Read the model definition and answer for the solid it produces. Units are mm, in the model's axes. A direction names the side the tool comes from. Coordinates: 2 decimals unless noted, no trailing zeros. Write each loop counter-clockwise with the first axis right and the second up, starting at its lowest first coordinate (ties: lowest second). Pieces come first, ordered by that corner, then holes.
(1) Find the intervals of material crossed by probe 1 along Y at (x, z) = (0, 3); probe 2 along Z at (x, y) = (3, -16); probe 3 along X at (y, z) = (1.5, 1), in increasing order.
(2) The mould has two halves that part along Y. Classify faces 4 (the cylindrical face through (-0.54, -2.44, 4.93)), 5 (the flat face through (9.737, 4.326, 5.988)), 6 (the flat face through (-0.3, -11.6, 5.7)): +Y half, -Y half, draft (parallel to the pull), parting line (faces both ways), or undercut.
(3) Which of the six approach directions +Z, -Z, +X, -X, +Y, -Y give full straight-line access (tool end or side, diameter ignored) to faces 1 (the flat face through (4.326, -9.737, 5.988)), 2 (the flat face through (4.364, 9.311, 3.982)), 3 (the flat face through (-4.364, -9.311, 3.982))?
(4) Section A-A on z = 7.25 is taken. Write down the section's boundary in (x, y), then the cut area to 3 significant figures.
(5) Section B-B on x = -5 is taken. Write down the section's boundary in (y, z), then the cut area to 3 significant figures.
(6) Given pin 1 (3 mm diameter, centred on x = 8.5, z = 6, fed in from -Y); pin 2 (1 mm diameter, centred on y = 8.5, z = 3, fed in from +X), each flat-ended and moving along its own axis, determine where each tip first touches the part or whether it passes through.
(7) Section C-C on x = -11 is taken. Write down the section's boundary in (y, z).
from build123d import *

# Parameters (mm, degrees)
SKETCH2_R           = 5.5
SKETCH2_R_2         = 2.5
BOSS_EXTRUDE1_DEPTH = 10
BOSS_EXTRUDE2_DEPTH = 0.75
CIRPATTERN1_COUNT   = 4


with BuildPart() as part:
    # Sketch2 → Boss-Extrude1 (new body)
    with BuildSketch(Plane.XY):
        Circle(SKETCH2_R)
        Circle(SKETCH2_R_2, mode=Mode.SUBTRACT)
    extrude(amount=BOSS_EXTRUDE1_DEPTH)

    # Sketch4 → Boss-Extrude2 (add, symmetric)
    with BuildSketch(Plane(origin=(0, -1.095927867, 4.746985116), x_dir=(0, 0.9743700647852367, 0.22495105434385892), z_dir=(0, 0.22495105434385892, -0.9743700647852367))):
        with BuildLine():
            Line((5.562035005, 4.289362297), (5.562035005, 15.338741246))
            ThreePointArc((5.562035005, 15.338741246), (1.102910343, 19.797865908), (-3.356214318, 15.338741246))
            Line((-3.356214318, 15.338741246), (-3.356214318, 3.072229714))
            ThreePointArc((-3.356214318, 3.072229714), (-1.450852963, 3.954597536), (0.520369242, 3.231231872))
            ThreePointArc((0.520369242, 3.231231872), (3.26034811, 2.716133916), (5.562035005, 4.289362297))
        make_face()
    boss_extrude2 = extrude(amount=BOSS_EXTRUDE2_DEPTH, both=True)

    # CirPattern1: Boss-Extrude2 ×4 about axis
    cirpattern1_axis = Axis((0, 0, 0), (0, 0, 1))
    for i in range(1, CIRPATTERN1_COUNT):
        add(boss_extrude2.rotate(cirpattern1_axis, i * 360 / CIRPATTERN1_COUNT))


solid = part.part
Response:
1. probe 1: y = -5.5 to -2.5, 2.5 to 5.5
1. probe 2: z = 4.92 to 6.46
1. probe 3: x = -5.29 to -2, 2 to 5.29
2. face 4: undercut
2. face 5: +Y half
2. face 6: draft
3. face 1: +Z, +X, -Y
3. face 2: -Z, +X, +Y
3. face 3: -Z, -X, -Y
4. outline: circle Ø11 at (0, 0); hole circle Ø5 at (0, 0)
4. area: 75.4 mm2
5. outline: (-4.49, 5.27) - (-2.29, 4.76) - (-2.29, 0) - (2.29, 0) - (2.29, 3.7) - (4.2, 3.26) - (4.53, 4.72) - (2.29, 5.24) - (2.29, 10) - (-2.29, 10) - (-2.29, 6.3) - (-4.15, 6.73) - close
5. area: 52.1 mm2
6. pin 1: stops at y = -4.53
6. pin 2: stops at x = 4.25
7. outline: (-4.49, 5.27) - (4.2, 3.26) - (4.53, 4.72) - (-4.15, 6.73) - close
